from build123d import *

# Parameters (mm, degrees)
SKETCH2_R           = 2.125
BOSS_EXTRUDE1_DEPTH = 8
FILLET2_R           = 0.5


with BuildPart() as part:
    # Sketch2 → Boss-Extrude1 (new body)
    with BuildSketch(Plane.XY):
        with BuildLine():
            Line((22.446269754, 6.096308238), (114.565217391, -3.976300301))
            ThreePointArc((114.565217391, -3.976300301), (118.976300301, -0.434782609), (115.434782609, 3.976300301))
            Line((115.434782609, 3.976300301), (23.315834971, 14.04890884))
            ThreePointArc((23.315834971, 14.04890884), (8.479435153, 11.762752399), (-3.226185769, 2.364682935))
            ThreePointArc((-3.226185769, 2.364682935), (-2.364682935, -3.226185769), (3.226185769, -2.364682935))
            ThreePointArc((3.226185769, -2.364682935), (11.702669886, 4.440815643), (22.446269754, 6.096308238))
        make_face()
        Circle(SKETCH2_R, mode=Mode.SUBTRACT)
        with Locations((115, 0)):
            Circle(SKETCH2_R, mode=Mode.SUBTRACT)
    extrude(amount=BOSS_EXTRUDE1_DEPTH)

    # Fillet2
    fillet2_edges = [part.edges().sort_by_distance(p)[0] for p in [
        (118.976300301, -0.434782609, 8),
        (69.37530879, 9.01260457, 8),
        (8.479435153, 11.762752399, 8),
        (-2.364682935, -3.226185769, 8),
        (11.702669886, 4.440815643, 8),
        (68.505743573, 1.060003968, 8),
    ]]
    fillet(fillet2_edges, radius=FILLET2_R)


solid = part.part
Check sheet for the modelled part. Datum: model origin and axes. Units: mm. A direction names the side the tool comes from. Round coordinates to 2 decimals unless told otherwise and drop trailing zeros. Loops run counter-clockwise (first coordinate to the right, second up) from the corner with the lowest first, then second, coordinate; pieces in that order, holes last. Notation, with made-up numbers: M 31,35.5 L 62,35.5 A5 cw 62,41.5 Z; hole C -5.5,22.25 d9. An arc over 180 degrees is marked long. One line per item, written item: value.
(1) Release check for a two-part mould opening along X. For faces 4 (the face through (1.142, 1.792, 3.944)), 5 (the face through (57, 5, 0)), 6 (the face through (70.02, 8.942, 3.698)) record: +X half, -X half, draft (parallel to the pull), parting line (faces both ways), or undercut.
Computed values:
face 4: undercut
face 5: draft
face 6: +X half
(2) Sectioned sample at A-A, the plane z = 2. Record the cut outline in (x, y) (3 decimals), then the cut area to 3 significant figures.
Computed values:
outline: M -3.226,2.365 A4 ccw 3.226,-2.365 A21 cw 22.446,6.096 L 114.565,-3.976 A4 ccw 115.435,3.976 L 23.316,14.049 A29 ccw Z; hole C 0,0 d4.25; hole C 115,0 d4.25
area: 973 mm^2
(3) Thickness scan on line 1 (Y direction, x = 115, z = 3) (3 decimals); line 2 (Y direction, x = 0, z = 2.5) (3 decimals); line 3 (Y direction, x = 13.5, z = 4.75). Record the ranges inside material, lowest first.
Computed values:
line 1: y = -4 to -2.125, 2.125 to 4.024
line 2: y = -4 to -2.125, 2.125 to 6.064
line 3: y = 5.14 to 13.44
(4) Depth check by flat-ended pin: pin 1 Ø1 at (x, y) = (68, 3.5) entering from -Z; pin 2 Ø1 at (x, z) = (14.5, 6.5) entering from +Y; pin 3 Ø2 at (x, z) = (66, 6) entering from +Y. Enter the tip coordinate at first touch or a pass-through.
Computed values:
pin 1: stops at z = 0
pin 2: stops at y = 13.76
pin 3: stops at y = 9.49
(5) Access from +Z, -Z, +X, -X, +Y, -Y to the whole of each face (thin tool, end or side, straight path). Record for faces 1 (the face through (67.86, 1.13, 3.7)), 2 (the face through (68.71, 8.94, 7.85)), 3 (the face through (69.17, 1.13, 7.85)).
Computed values:
face 1: +Z, -Z, -Y
face 2: +Z, +X, +Y
face 3: +Z, -Y
(6) Sectioned sample at B-B, the plane y = -1. Count the separate pieces of the cut face and the enclosed holes in it, then the cut area to 3 significant figures.
Computed values:
separate pieces: 4
enclosed holes: 0
area: 257 mm^2
